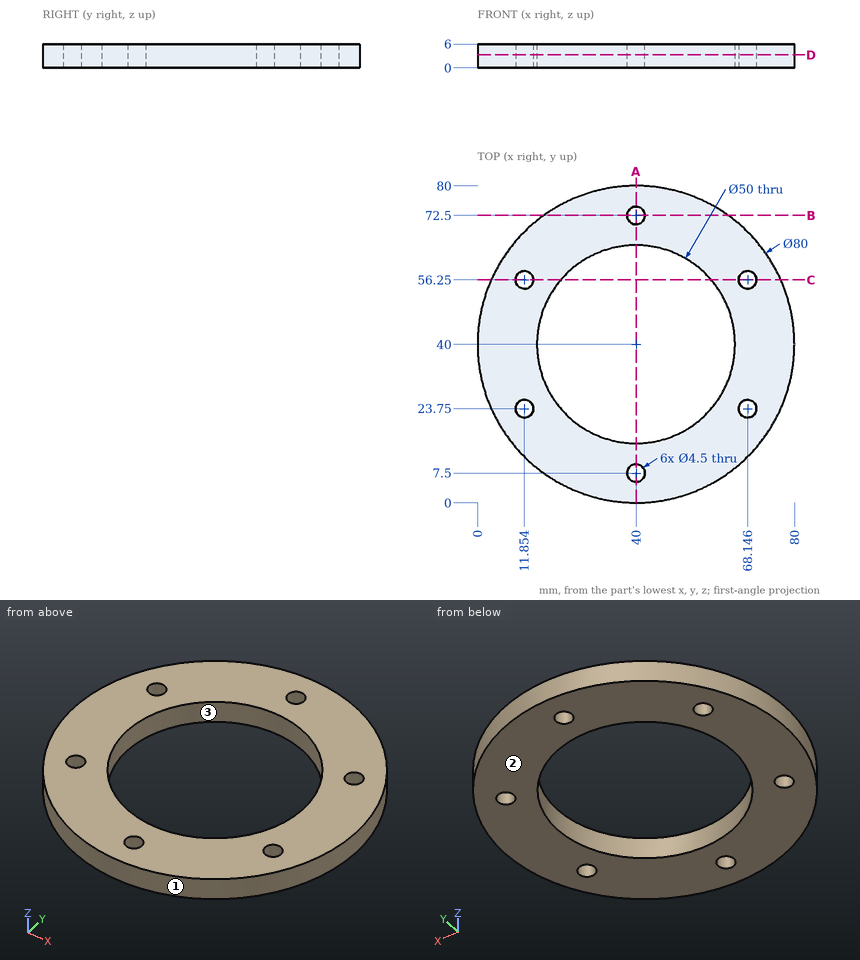
The drawing under review shows one solid part. Ordinate dimensions are in mm from its lowest x, y, z. Coordinates: 2 decimals unless noted, no trailing zeros. Write each loop counter-clockwise with the first axis right and the second up, starting at its lowest first coordinate (ties: lowest second). Pieces come first, ordered by that corner, then holes. Notation, with made-up numbers: (17.5, 76.25) - (34.5, 76.25) arc R9 cw to (34.5, 80.25) - close; hole circle Ø6 at (-40, 34.25). An arc over 180 degrees is marked (long way). Use one line per item in the form item = value.
Q1. For probe 1 along Y at (x, z) = (40, 4.4); probe 2 along Y at (x, z) = (39, 4) (1 decimal); probe 3 along X at (y, z) = (24, 5.2), list the stretches that pass through material, from the lowest coordinate up.
Taken from the geometry:
probe_1 = 0 to 5.25, 9.75 to 15, 65 to 70.25, 74.75 to 80
probe_2 = 0 to 5.5, 9.5 to 15, 65 to 70.5, 74.5 to 80
probe_3 = 3.34 to 9.62, 14.09 to 20.79, 59.21 to 65.91, 70.38 to 76.66
Q2. Consider section C-C (y = 56.25). Write out the cut boundary in (x, z), plus the area to 3 significant figures.
Taken from the geometry:
outline = (3.45, 0) - (9.6, 0) - (9.6, 6) - (3.45, 6) - close; (14.1, 0) - (21, 0) - (21, 6) - (14.1, 6) - close; (59, 0) - (65.9, 0) - (65.9, 6) - (59, 6) - close; (70.4, 0) - (76.55, 0) - (76.55, 6) - (70.4, 6) - close
area = 157 mm^2
Q3. Consider section A-A (x = 40). Write out the cut boundary in (y, z), plus the area to 3 significant figures.
Taken from the geometry:
outline = (0, 0) - (5.25, 0) - (5.25, 6) - (0, 6) - close; (9.75, 0) - (15, 0) - (15, 6) - (9.75, 6) - close; (65, 0) - (70.25, 0) - (70.25, 6) - (65, 6) - close; (74.75, 0) - (80, 0) - (80, 6) - (74.75, 6) - close
area = 126 mm^2
Q4. Consider section D-D (z = 3.25). Write out the cut boundary in (x, y), plus the area to 3 significant figures.
Taken from the geometry:
outline = circle Ø80 at (40, 40); hole circle Ø4.5 at (11.85, 23.75); hole circle Ø4.5 at (11.85, 56.25); hole circle Ø50 at (40, 40); hole circle Ø4.5 at (40, 7.5); hole circle Ø4.5 at (40, 72.5); hole circle Ø4.5 at (68.15, 23.75); hole circle Ø4.5 at (68.15, 56.25)
area = 2,970 mm^2
Q5. The part is to be moulded in two halves that separate along X. For the marked faces 1, 2 and 3, say which applies: +X half, -X half, draft (parallel to the pull), parting line (faces both ways), or undercut.
Taken from the geometry:
face_1 = parting line
face_2 = draft
face_3 = undercut
Q6. Consider section B-B (y = 72.5). Write out the cut boundary in (x, z), plus the area to 3 significant figures.
Taken from the geometry:
outline = (16.68, 0) - (37.75, 0) - (37.75, 6) - (16.68, 6) - close; (42.25, 0) - (63.32, 0) - (63.32, 6) - (42.25, 6) - close
area = 253 mm^2
Q7. Insertion check: pin 1 Ø6 at (x, y) = (22.5, 54.5) entering from -Z; pin 2 Ø1.5 at (x, z) = (59, 1.5) entering from +Y. Each pin has a flat end and moves straight along its axis. Give the tip position at first contact, or say it passes through.
Taken from the geometry:
pin_1 = 0
pin_2 = 75.59
